from build123d import *

# Parameters (mm, degrees)
SKETCH1_R           = 1.6
BOSS_EXTRUDE1_DEPTH = 4


with BuildPart() as part:
    # Sketch1 → Boss-Extrude1 (new body)
    with BuildSketch(Plane(origin=(0, 0, 0), x_dir=(-1, 0, 0), z_dir=(0, 0, 1))):
        Polygon((-20, 40), (20, 40), (20, 32.5), (36.828427125, 32.5), (36.828427125, 7.5), (20, 7.5), (20, 0), (-20, 0), (-20, 7.5), (-15.171572875, 7.5), (-15.171572875, 32.5), (-20, 32.5), align=None)
        with Locations(Location((-7.6, 31, 0), (0, 0, 180))):
            Circle(SKETCH1_R, mode=Mode.SUBTRACT)
        with Locations((7.6, 31)):
            Circle(SKETCH1_R, mode=Mode.SUBTRACT)
        with Locations(Location((0, 2, 0), (0, 0, 180))):
            Circle(SKETCH1_R, mode=Mode.SUBTRACT)
    extrude(amount=BOSS_EXTRUDE1_DEPTH)


solid = part.part
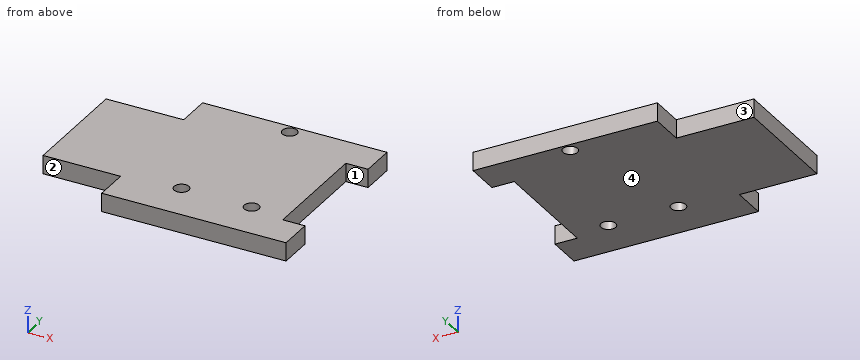
For this review, take the finished solid that the model builds, in its own axes (mm). Face numbers are marked on the shaded views. A direction names the side the tool comes from. Round coordinates to 2 decimals unless told otherwise and drop trailing zeros. Write each loop counter-clockwise with the first axis right and the second up, starting at its lowest first coordinate (ties: lowest second). Pieces come first, ordered by that corner, then holes. Notation, with made-up numbers: (3.5, 12) - (7.5, 12) arc R21 ccw to (7.5, 37) - close; hole circle Ø3 at (64.5, -13.75). An arc over 180 degrees is marked (long way). Write item = value, one per line. Start each with the question number.
1. For the marked faces 1, 2, 3 and 4, list the 3-axis set-ups (+Z, -Z, +X, -X, +Y, -Y) from which the entire face can be reached by the end or side of a thin tool; tool diameter is ignored.
2. Consider section A-A on z = 2.4. State the section outline as (x, y) points, plus the area to 3 significant figures.
3. Consider section D-D on y = -6.5. State the section outline as (x, z) points.
4. Consider section C-C on y = -2. State the section outline as (x, z) points, plus the area to 3 significant figures.
5. Consider section B-B on x = 0. State the section outline as (y, z) points, plus the area to 3 significant figures.
6. For pin 1 Ø2.5 at (x, y) = (7.6, -31) entering from -Z; pin 2 Ø2 at (x, y) = (1.5, -21.5) entering from -Z; pin 3 Ø2 at (y, z) = (-4.5, 2) entering from -X; pin 4 Ø1.2 at (x, z) = (-25.5, 2.5) entering from +Y, all flat-tipped, find the tip position at first contact; note any pin that passes through.
7. Wall thickness on L1, parallel to Y at x = 7.6, z = 1.4; L2, parallel to Y at x = 0, z = 3; L3, parallel to X at y = -8.5, z = 3.3: over which ranges is each line inside the solid? List them lowest first.
Evaluation:
q1.face_1 = +Z, -Z, +X
q1.face_2 = +Z, -Z, -X, -Y
q1.face_3 = +Z, -Z, -X, +Y
q1.face_4 = -Z, +X, -X, +Y, -Y
q2.outline = (-36.83, -32.5) - (-20, -32.5) - (-20, -40) - (20, -40) - (20, -32.5) - (15.17, -32.5) - (15.17, -7.5) - (20, -7.5) - (20, 0) - (-20, 0) - (-20, -7.5) - (-36.83, -7.5) - close; hole circle Ø3.2 at (-7.6, -31); hole circle Ø3.2 at (0, -2); hole circle Ø3.2 at (7.6, -31)
q2.area = 1,880 mm2
q3.outline = (-20, 0) - (20, 0) - (20, 4) - (-20, 4) - close
q4.outline = (-20, 0) - (-1.6, 0) - (-1.6, 4) - (-20, 4) - close; (1.6, 0) - (20, 0) - (20, 4) - (1.6, 4) - close
q4.area = 147 mm2
q5.outline = (-40, 0) - (-3.6, 0) - (-3.6, 4) - (-40, 4) - close; (-0.4, 0) - (0, 0) - (0, 4) - (-0.4, 4) - close
q5.area = 147 mm2
q6.pin_1 = through
q6.pin_2 = 0
q6.pin_3 = -20
q6.pin_4 = -7.5
q7.L1 = -40 to -32.6, -29.4 to 0
q7.L2 = -40 to -3.6, -0.4 to 0
q7.L3 = -36.83 to 15.17
